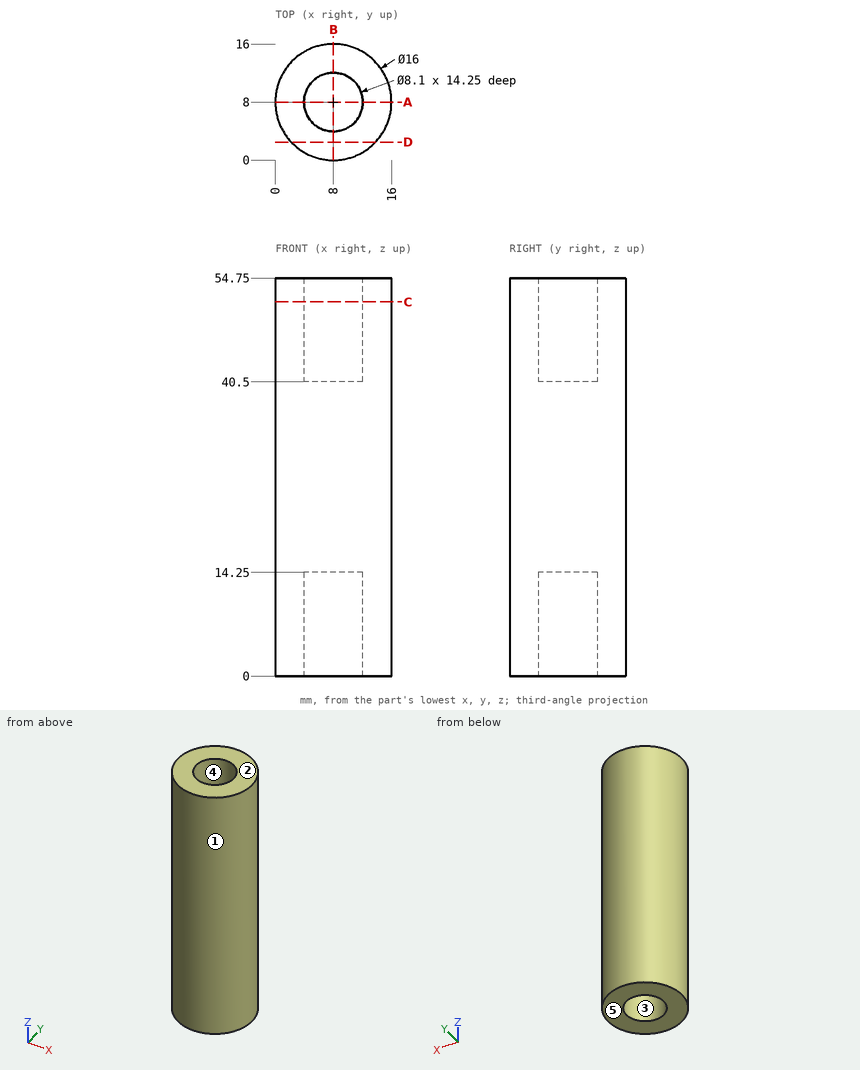
Input: dimensioned drawing with shaded views. Units: mm. Origin: part minimum x, y, z. A direction names the side the tool comes from. Round coordinates to 2 decimals unless told otherwise and drop trailing zeros. Order: outer loops, then holes, each group sorted by start corner. A loop starts at its lowest first (then second) coordinate and runs counter-clockwise, first axis right, second up. Notation, with made-up numbers: (12, 2) -> (19, 2) arc R23 ccw to (19, 18) -> close; hole circle Ø2 at (64, 10). An arc over 180 degrees is marked (long way). One line per item, written item: value. Start each with the question number.
Q1. Section query D-D (y = 2.5). Return the cut outline in (x, z).
Q2. Draft query along X for the marked faces 1, 2 and 3. Return one class per face: pulls with the +X half, pulls with the -X half, needs draft (parallel to the pull), parting line crosses it, or undercut.
Q3. Section query C-C (z = 51.5). Return the cut outline in (x, y), plus the area to 3 significant figures.
Q4. Pin query (flat end, axial travel): pin 1 (1.5 mm diameter, centred on x = 6.5, y = 10, fed in from +Z); pin 2 (1 mm diameter, centred on x = 14, z = 25.5, fed in from -Y); pin 3 (1.5 mm diameter, centred on x = 7, z = 19, fed in from +Y). Return the tip coordinate at first contact, or that it passes through.
Q5. Section query A-A (y = 8). Return the cut outline in (x, z).
Q6. Access query for the marked faces 4 and 5. Directions: +Z, -Z, +X, -X, +Y, -Y. A direction counts if a zero-diameter tool reaches every point of the face in a straight line with its end or side. Return the directions, or none.
Q7. Material intervals for probe 1 along Y at (x, z) = (8, 10.5); probe 2 along Z at (x, y) = (9.25, 7.25); probe 3 along X at (y, z) = (7.75, 7), sorted ascending.
Findings below:
1. outline: (2.19, 0) -> (13.81, 0) -> (13.81, 54.75) -> (2.19, 54.75) -> close
2. face 1: parting line crosses it
2. face 2: needs draft
2. face 3: undercut
3. outline: circle Ø16 at (8, 8); hole circle Ø8.1 at (8, 8)
3. area: 150 mm²
4. pin 1: z = 40.5
4. pin 2: y = 2.19
4. pin 3: y = 16
5. outline: (0, 0) -> (3.95, 0) -> (3.95, 14.25) -> (12.05, 14.25) -> (12.05, 0) -> (16, 0) -> (16, 54.75) -> (12.05, 54.75) -> (12.05, 40.5) -> (3.95, 40.5) -> (3.95, 54.75) -> (0, 54.75) -> close
6. face 4: +Z
6. face 5: -Z, +X, -X, +Y, -Y
7. probe 1: 0 to 3.95, 12.05 to 16
7. probe 2: 14.25 to 40.5
7. probe 3: 0 to 3.96, 12.04 to 16
